Build history of the part. All positions in model axes, mm. A direction names the side the tool comes from. Round coordinates to 2 decimals unless told otherwise and drop trailing zeros. Loops run counter-clockwise (first coordinate to the right, second up) from the corner with the lowest first, then second, coordinate; pieces in that order, holes last. Notation, with made-up numbers: (-38, -13.5) - (-27, -13.5) arc R4 ccw to (-27, -6.5) - close; hole circle Ø1 at (69, 33.25). An arc over 180 degrees is marked (long way). Use a Markdown table: item, result.
from build123d import *

# Parameters (mm, degrees)
F0_W     = 40
F0_H     = 10
F0_R     = 3.75
F1_DEPTH = 3.5
F3_DEPTH = 2


# Not quite as in the source:
# - a pattern or mirror of a feature is missing from the dataset's text; its kind, count and spacing are read off the source's solid


with BuildPart() as f1:
    # F0 (on Front) → F1 (new body)
    with BuildSketch(Plane.XZ):
        with Locations((20, 7.299159328)):
            Rectangle(F0_W, F0_H)
        with Locations((20, 7.299159328)):
            Circle(F0_R, mode=Mode.SUBTRACT)
    extrude(amount=F1_DEPTH)

    # F2 (on face) → F3 (cut)
    with BuildSketch(Plane.XZ.offset(3.5)):
        with BuildLine():
            ThreePointArc((17.5055060633, 4.499159328), (16.25, 7.299159328), (17.5055060633, 10.099159328))
            Line((17.5055060633, 10.099159328), (4.8898644293, 9.4033881317))
            ThreePointArc((4.8898644293, 9.4033881317), (3.5473694307, 8.7811462961), (3, 7.4064228951))
            Line((3, 7.4064228951), (3, 7.1918957609))
            ThreePointArc((3, 7.1918957609), (3.5473694307, 5.8171723599), (4.8898644293, 5.1949305243))
            Line((4.8898644293, 5.1949305243), (17.5055060633, 4.499159328))
        make_face()
    f3 = extrude(amount=-F3_DEPTH, mode=Mode.SUBTRACT)

    # F3_copies: F3 across plane
    add(f3.mirror(Plane(origin=(20, 0, 0), x_dir=(0, 0, 1), z_dir=(1, 0, 0))), mode=Mode.SUBTRACT)


solid = f1.part
Q1. Cut at B-B, the plane x = 20. List the corners of the cut face in (y, z).
Results found:
| item | result |
|---|---|
| outline | (-3.5, 2.3) - (0, 2.3) - (0, 3.55) - (-3.5, 3.55) - close; (-3.5, 11.05) - (0, 11.05) - (0, 12.3) - (-3.5, 12.3) - close |
Q2. Pull direction X, two halves, no side cores. Call faces 1 (the face through (40, -2, 7)), 2 (the face through (20, -2, 12.299)), 3 (the face through (28.89, -2.51, 4.85)): pulls with the +X half, pulls with the -X half, needs draft (parallel to the pull), parting line crosses it, or undercut.
Results found:
| item | result |
|---|---|
| face 1 | pulls with the +X half |
| face 2 | needs draft |
| face 3 | undercut |
Q3. Cut at D-D, the plane x = 28. List the corners of the cut face in (y, z), plus the area to 3 significant figures.
Results found:
| item | result |
|---|---|
| outline | (-3.5, 2.3) - (0, 2.3) - (0, 12.3) - (-3.5, 12.3) - (-3.5, 9.8) - (-1.5, 9.8) - (-1.5, 4.8) - (-3.5, 4.8) - close |
| area | 25.0 mm2 |
Q4. Cut at A-A, the plane y = -2. List the corners of the cut face in (x, z).
Results found:
| item | result |
|---|---|
| outline | (0, 2.3) - (40, 2.3) - (40, 12.3) - (0, 12.3) - close; hole (3, 7.19) arc R2 ccw to (4.89, 5.19) - (17.51, 4.5) arc R3.75 ccw to (22.49, 4.5) - (35.11, 5.19) arc R2 ccw to (37, 7.19) - (37, 7.41) arc R2 ccw to (35.11, 9.4) - (22.49, 10.1) arc R3.75 ccw to (17.51, 10.1) - (4.89, 9.4) arc R2 ccw to (3, 7.41) - close |
Q5. Probe line 1 (Z direction, x = 20, y = -2.3); line 2 (Y direction, x = 27, z = 9); line 3 (X direction, y = -0.2, z = 10.75). List the from-to ranges inside material, lowest first.
Results found:
| item | result |
|---|---|
| line 1 | z = 2.3 to 3.55, 11.05 to 12.3 |
| line 2 | y = -1.5 to 0 |
| line 3 | x = 0 to 18.53, 21.47 to 40 |
Q6. Cut at C-C, the plane z = 5.75. List the corners of the cut face in (x, y).
Results found:
| item | result |
|---|---|
| outline | (0, -3.5) - (3.61, -3.5) - (3.61, -1.5) - (16.58, -1.5) - (16.58, 0) - (0, 0) - close; (23.42, -1.5) - (36.39, -1.5) - (36.39, -3.5) - (40, -3.5) - (40, 0) - (23.42, 0) - close |
Q7. Drop flat-ended pins along their axis: pin 1 (1 mm diameter, centred on y = -0.5, z = 8, fed in from -X); pin 2 (3 mm diameter, centred on x = 30, z = 8, fed in from -Y). Give the stop position or say it passes through.
Results found:
| item | result |
|---|---|
| pin 1 | stops at x = 0 |
| pin 2 | stops at y = -1.5 |
Q8. Which spindle directions (+Z, -Z, +X, -X, +Y, -Y) get a long thin tool onto all of the face, cutting with end or side? Do faces 4 (the face through (36.438, -2.514, 8.796)), 5 (the face through (23.577, -1.337, 8.426)). Say none if no direction does.
Results found:
| item | result |
|---|---|
| face 4 | -Y |
| face 5 | +Y, -Y |
